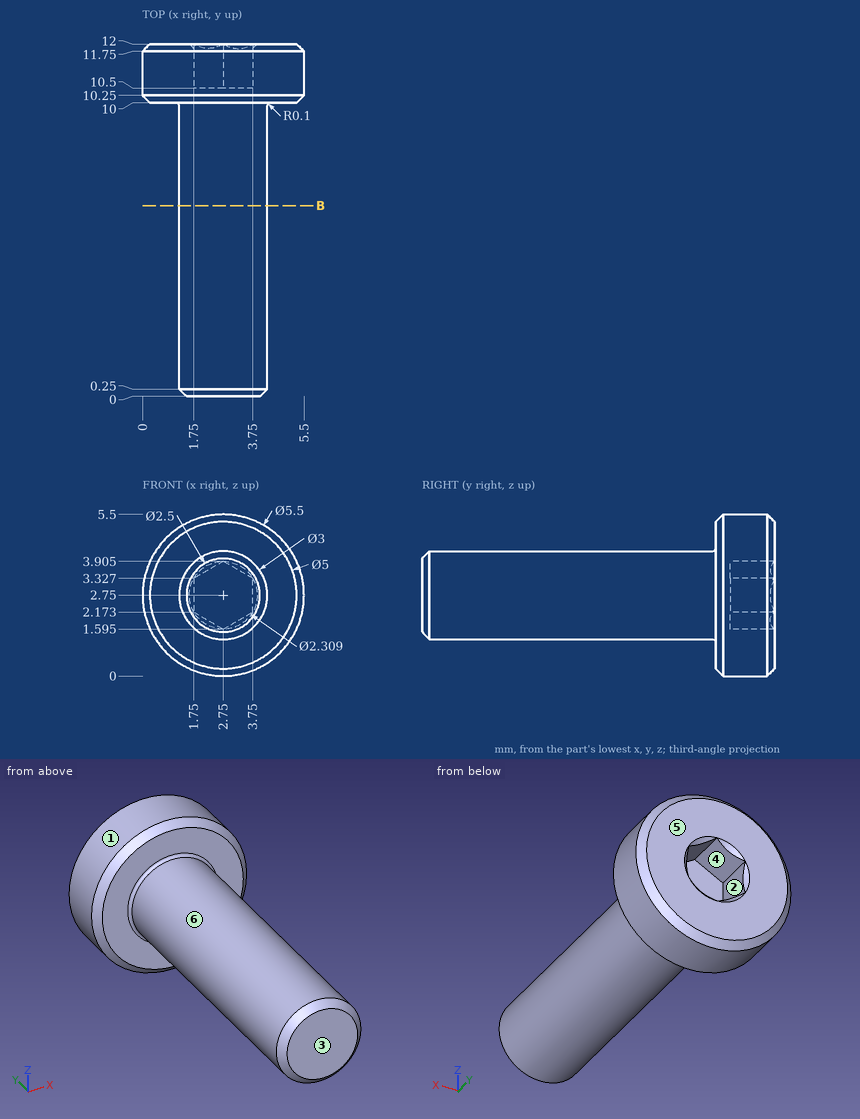
Geometry check sheet. Reference: drawing and pictorial views, mm from the part's lowest x, y, z. A direction names the side the tool comes from. Coordinates: 2 decimals unless noted, no trailing zeros. Order: outer loops, then holes, each group sorted by start corner. A loop starts at its lowest first (then second) coordinate and runs counter-clockwise, first axis right, second up. Notation, with made-up numbers: M 44,-23.75 L 93,-23.75 A21 ccw 93,-2.75 Z; hole C -7.5,9.5 d9. An arc over 180 degrees is marked long. Write each question's results on one line, items separated by ' | '. Start each with the question number.
1. Access from +Z, -Z, +X, -X, +Y, -Y to the whole of each face (thin tool, end or side, straight path). Record for the marked faces 4, 5 and 6.
2. Cross-section at B-B on y = 6.5. Record the cut outline in (x, z).
3. Go/stop test with flat-tipped pins: P1, Ø2, axis at x = 5, y = 8, coming from the -Z side; P2, Ø1.5, axis at x = 0.5, z = 4.5, coming from the -Y side; P3, Ø1, axis at x = 3, y = 4.5, coming from the -Z side; P4, Ø1.5, axis at x = 2.5, z = 1.5, coming from the -Y side. Record where each tip stops, or that it passes through.
4. Mould release check, pull along X, two halves, no side actions. Record for the marked faces 1, 2 and 3: +X half, -X half, draft (parallel to the pull), parting line (faces both ways), or undercut.
5. Material ranges on probe 1 along Y at (x, z) = (5.2, 3.05); probe 2 along Y at (x, z) = (2.05, 2.2); probe 3 along X at (y, z) = (10.75, 1.75) (1 decimal), recorded low to high.
Checks:
1) face 4: +Y | face 5: +Z, -Z, +X, -X, +Y | face 6: -Y
2) outline: C 2.75,2.75 d3
3) P1: stops at z = 1.92 | P2: stops at y = 10 | P3: stops at z = 1.25 | P4: stops at y = 0
4) face 1: parting line | face 2: undercut | face 3: draft
5) probe 1: y = 10 to 12 | probe 2: y = 0 to 10.5 | probe 3: x = 0.2 to 2.5, 3 to 5.3
